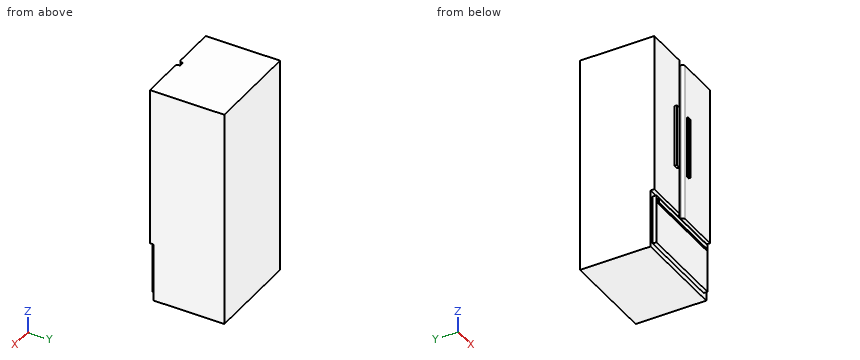
from build123d import *

# Parameters (mm, degrees)
F0_W      = 762
F0_H      = 563.88
F1_DEPTH  = 1752.6
F2_W      = 696.7959
F2_H      = 392.960511
F3_DEPTH  = 30.48
F4_W      = 361.621648
F4_H      = 1283.220664
F4_W_2    = 362.307822
F5_DEPTH  = 30.48
F6_R      = 22.075569
F7_W      = 35.273701
F7_H      = 499.968111
F8_DEPTH  = 18.288
F9_W      = 27.252704
F9_H      = 490.54879
F10_DEPTH = 12.192
F11_W     = 660.017151
F11_H     = 33.723503
F12_DEPTH = 12.192


with BuildPart() as f1:
    # F0 (on Top) → F1 (new body)
    with BuildSketch(Plane.XY):
        with Locations((381, -281.94)):
            Rectangle(F0_W, F0_H)
    extrude(amount=F1_DEPTH)

    # F2 (on face) → F3 (join)
    with BuildSketch(Plane.XZ.offset(563.88)):
        with Locations((377.334675, 238.608349)):
            Rectangle(F2_W, F2_H)
    extrude(amount=F3_DEPTH)

    # F4 (on face) → F5 (join)
    with BuildSketch(Plane.XZ.offset(563.88)):
        with Locations((180.810824, 1110.989668)):
            Rectangle(F4_W, F4_H)
        with Locations((580.846089, 1110.989668)):
            Rectangle(F4_W_2, F4_H)
    extrude(amount=F5_DEPTH)

    # F6
    f6_edges = [f1.edges().sort_by_distance(p)[0] for p in [
        (361.621648, -594.36, 1110.989668),
        (399.692178, -594.36, 1110.989668),
    ]]
    fillet(f6_edges, radius=F6_R)

    # F7 (on face) → F8 (join)
    with BuildSketch(Plane.XZ.offset(594.36)):
        with Locations((293.69308, 1080.406278)):
            Rectangle(F7_W, F7_H)
    extrude(amount=F8_DEPTH)

    # F9 (on face) → F10 (join)
    with BuildSketch(Plane.XZ.offset(594.36)):
        with Locations((456.993356, 1084.997684)):
            Rectangle(F9_W, F9_H)
    extrude(amount=F10_DEPTH)

    # F11 (on face) → F12 (join)
    with BuildSketch(Plane.XZ.offset(594.36)):
        with Locations((376.0538, 397.549763)):
            Rectangle(F11_W, F11_H)
    extrude(amount=F12_DEPTH)


solid = f1.part
CAD build for the part. Positions are in the model's coordinates, mm. Round coordinates to 2 decimals unless told otherwise and drop trailing zeros. Order: outer loops, then holes, each group sorted by start corner. A loop starts at its lowest first (then second) coordinate and runs counter-clockwise, first axis right, second up. Notation, with made-up numbers: (0.25, 85.25) - (9.25, 85.25) arc R13 ccw to (9.25, 99.25) - close; hole circle Ø5 at (44, 63.5). An arc over 180 degrees is marked (long way). Return JSON: item names as keys, results as strings.
(1) Wall check: probe 1 along Y at (x, z) = (191.5, 1195.5); probe 2 along Y at (x, z) = (365.5, 1525.5). Give the ranges that are in metal, low to high. Write a range as from..to.
Answer key:
{"probe 1": "y = -594.36..0", "probe 2": "y = -563.88..0"}
(2) Cut at B-B (z = 1486). Give the cut face in (x, y).
Answer key:
{"outline": "(0, -594.36) - (339.55, -594.36) arc R22.08 ccw to (361.62, -572.28) - (361.62, -563.88) - (399.69, -563.88) - (399.69, -572.28) arc R22.08 ccw to (421.77, -594.36) - (762, -594.36) - (762, 0) - (0, 0) - close"}
(3) Pin check, flat tips, straight feed: pin 1 Ø6 at (x, y) = (454, -600.5) entering from +Z; pin 2 Ø5.5 at (y, z) = (-607.5, 990) entering from +X; pin 3 Ø10 at (y, z) = (-603.5, 396.5) entering from +X. Stop position of each tip, or through.
Answer key:
{"pin 1": "stops at z = 1330.27", "pin 2": "stops at x = 470.62", "pin 3": "stops at x = 706.06"}
(4) Cut at C-C (z = 1005). Give the cut face in (x, y), then the cut area to 3 significant figures.
Answer key:
{"outline": "(0, -594.36) - (276.06, -594.36) - (276.06, -612.65) - (311.33, -612.65) - (311.33, -594.36) - (339.55, -594.36) arc R22.08 ccw to (361.62, -572.28) - (361.62, -563.88) - (399.69, -563.88) - (399.69, -572.28) arc R22.08 ccw to (421.77, -594.36) - (443.37, -594.36) - (443.37, -606.55) - (470.62, -606.55) - (470.62, -594.36) - (762, -594.36) - (762, 0) - (0, 0) - close", "area": "453,000 mm^2"}
(5) Cut at A-A (x = 190). Give the cut face in (y, z), then the cut area to 3 significant figures.
Answer key:
{"outline": "(-606.55, 380.69) - (-594.36, 380.69) - (-594.36, 42.13) - (-563.88, 42.13) - (-563.88, 0) - (0, 0) - (0, 1752.6) - (-594.36, 1752.6) - (-594.36, 469.38) - (-563.88, 469.38) - (-563.88, 435.09) - (-594.36, 435.09) - (-594.36, 414.41) - (-606.55, 414.41) - close", "area": "1,040,000 mm^2"}
(6) Cut at D-D (z = 208). Give the cut face in (x, y), then the cut area to 3 significant figures.
Answer key:
{"outline": "(0, -563.88) - (28.94, -563.88) - (28.94, -594.36) - (725.73, -594.36) - (725.73, -563.88) - (762, -563.88) - (762, 0) - (0, 0) - close", "area": "451,000 mm^2"}
